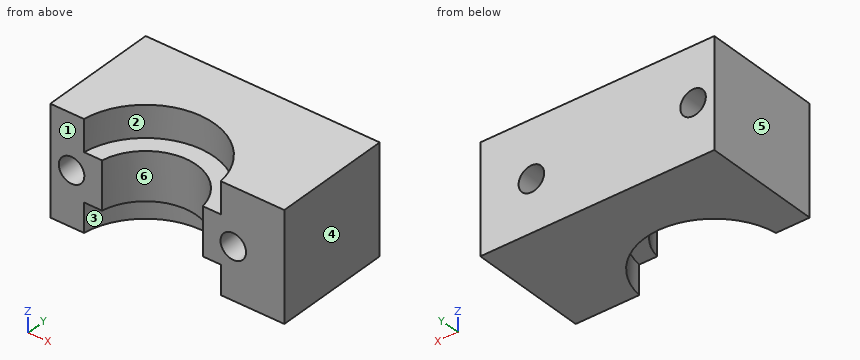
```python
from build123d import *

# Parameters (mm, degrees)
SKETCH1_W           = 24
SKETCH1_H           = 12.7
BOSS_EXTRUDE1_DEPTH = 15
SKETCH2_R           = 6
CUT_EXTRUDE1_DEPTH  = 15
SKETCH3_R           = 8.1
CUT_EXTRUDE2_DEPTH  = 3.7
CUT_EXTRUDE3_START  = -3.4
SKETCH5_R           = 8.1
CUT_EXTRUDE3_DEPTH  = 3.4
SKETCH6_W           = 24
SKETCH6_H           = 12.7
CUT_EXTRUDE4_DEPTH  = 1
SKETCH7_R           = 1.5
CUT_EXTRUDE5_DEPTH  = 22
SKETCH8_W           = 12.7
SKETCH8_H           = 14
BOSS_EXTRUDE2_DEPTH = 3.5


with BuildPart() as part:
    # Sketch1 → Boss-Extrude1 (new body)
    with BuildSketch(Plane(origin=(0, 0, 0), x_dir=(1, 0, 0), z_dir=(0, 1, 0))):
        with Locations((-12, 6.35)):
            Rectangle(SKETCH1_W, SKETCH1_H)
    extrude(amount=BOSS_EXTRUDE1_DEPTH)

    # Sketch2 → Cut-Extrude1 (cut)
    with BuildSketch(Plane.XY):
        with Locations((-12, 0)):
            Circle(SKETCH2_R)
    extrude(amount=-CUT_EXTRUDE1_DEPTH, mode=Mode.SUBTRACT)

    # Sketch3 → Cut-Extrude2 (cut)
    with BuildSketch(Plane.XY):
        with Locations((-12, 0)):
            Circle(SKETCH3_R)
    extrude(amount=-CUT_EXTRUDE2_DEPTH, mode=Mode.SUBTRACT)

    # Sketch5 → Cut-Extrude3 (cut)
    with BuildSketch(Plane(origin=(0, 0, -12.7), x_dir=(-1, 0, 0), z_dir=(0, 0, -1)).offset(CUT_EXTRUDE3_START)):
        with Locations((12, 0)):
            Circle(SKETCH5_R)
    extrude(amount=CUT_EXTRUDE3_DEPTH, mode=Mode.SUBTRACT)

    # Sketch6 → Cut-Extrude4 (cut)
    with BuildSketch(Plane.XZ):
        with Locations((-12, -6.35)):
            Rectangle(SKETCH6_W, SKETCH6_H)
    extrude(amount=-CUT_EXTRUDE4_DEPTH, mode=Mode.SUBTRACT)

    # Sketch7 → Cut-Extrude5 (cut)
    with BuildSketch(Plane.XZ.offset(-1)):
        with Locations(Location((-21.5, -6.35, 0), (0, 0, 270))):
            Circle(SKETCH7_R)
        with Locations(Location((-2.5, -6.65, 0), (0, 0, 270))):
            Circle(SKETCH7_R)
    extrude(amount=-CUT_EXTRUDE5_DEPTH, mode=Mode.SUBTRACT)

    # Sketch8 → Boss-Extrude2 (add)
    with BuildSketch(Plane(origin=(0, 0, 0), x_dir=(0, 0, -1), z_dir=(1, 0, 0))):
        with Locations((6.35, 8)):
            Rectangle(SKETCH8_W, SKETCH8_H)
    extrude(amount=BOSS_EXTRUDE2_DEPTH)


solid = part.part
```
The model under review builds one solid part; all positions refer to its coordinate system, in mm. Face numbers are marked on the shaded views. A direction names the side the tool comes from. Round coordinates to 2 decimals unless told otherwise and drop trailing zeros. Loops run counter-clockwise (first coordinate to the right, second up) from the corner with the lowest first, then second, coordinate; pieces in that order, holes last.
1) The part is to be moulded in two halves that separate along X. For the marked faces 4, 5 and 6, say which applies: pulls with the +X half, pulls with the -X half, needs draft (parallel to the pull), parting line crosses it, or undercut.
Values follow:
face 4: pulls with the +X half
face 5: pulls with the -X half
face 6: undercut
2) Tool access review of the marked faces 1, 2 and 3: name each direction out of +Z, -Z, +X, -X, +Y, -Y from which nothing blocks a thin tool from reaching the whole face with its end or side.
Values follow:
face 1: +Z, -Z, +X, -X, -Y
face 2: +Z, -Y
face 3: -Z, -Y
3) Consider section C-C on z = -6.75. State the section outline as (x, y) points, then the cut area to 3 significant figures.
Values follow:
outline: (-24, 1) - (-22.95, 1) - (-22.95, 15) - (-24, 15) - close; (-20.05, 1) - (-17.92, 1) arc R6 cw to (-6.08, 1) - (-4, 1) - (-4, 15) - (-20.05, 15) - close; (-1, 1) - (3.5, 1) - (3.5, 15) - (-1, 15) - close
area: 258 mm2
4) Clearance check with a flat-ended pin moving along its axis: P1, Ø2, axis at x = -11.5, y = 3.5, coming from the +Z side. State where the tip first meets the part, or that it passes through.
Values follow:
P1: passes through
5) Wall thickness on line 1 along X through (y, z) = (11.5, -5.75); line 2 along X through (y, z) = (5.5, -6.35); line 3 along X through (y, z) = (8, -6.35): over which ranges is each line inside the solid? List them lowest first.
Values follow:
line 1: x = -24 to -22.87, -20.13 to -3.7, -1.3 to 3.5
line 2: x = -24 to -23, -20 to -14.4, -9.6 to -3.97, -1.03 to 3.5
line 3: x = -24 to -23, -20 to -3.97, -1.03 to 3.5
6) Consider section D-D on z = -0.75. State the section outline as (x, y) points.
Values follow:
outline: (-24, 1) - (-20.04, 1) arc R8.1 cw to (-3.96, 1) - (3.5, 1) - (3.5, 15) - (-24, 15) - close
7) Consider section B-B on x = -2.5. State the section outline as (y, z) points.
Values follow:
outline: (1, -12.7) - (15, -12.7) - (15, -8.15) - (1, -8.15) - close; (1, -5.15) - (15, -5.15) - (15, 0) - (1, 0) - close
8) Consider section A-A on y = 12.25. State the section outline as (x, z) points.
Values follow:
outline: (-24, -12.7) - (3.5, -12.7) - (3.5, 0) - (-24, 0) - close; hole circle Ø3 at (-21.5, -6.35); hole circle Ø3 at (-2.5, -6.65)
